Could you check a few things on this model? Use its own coordinates, in mm. Face numbers are marked on the shaded views. Give positions to 0.01 mm unless a question says otherwise; leave off trailing zeros. Write each loop counter-clockwise with the first axis right and the second up, starting at its lowest first coordinate (ties: lowest second). Pieces come first, ordered by that corner, then holes. Notation, with made-up numbers: (-9.75, 36) - (40.25, 36) arc R24 cw to (40.25, 48) - close; hole circle Ø5 at (71, -2). An arc over 180 degrees is marked (long way). Answer as a JSON object with one key per item and string values. Group by question number.
```python
from build123d import *

# Parameters (mm, degrees)
F3_DEPTH = 3.81
F4_R     = 1.27


# Not quite as in the source:
# - the program builds the solid bodies; features that only make, move or delete a surface that nothing else refers to are left out


with BuildPart() as f3:
    # F2 (on Front) → F3 (new body, symmetric)
    with BuildSketch(Plane.XZ):
        Polygon((67.4008423153, 47.9680152879), (42.0008423153, 47.9680152879), (33.6273413479, 18.6607656464), (59.0273413479, 18.6607656464), align=None)
    extrude(amount=F3_DEPTH, both=True)

    # F4
    f4_edges = [f3.edges().sort_by_distance(p)[0] for p in [
        (54.700842, -3.81, 47.968015),
        (63.214092, -3.81, 33.31439),
        (46.327341, -3.81, 18.660766),
        (63.214092, 3.81, 33.31439),
        (54.700842, 3.81, 47.968015),
        (46.327341, 3.81, 18.660766),
        (67.400842, 0, 47.968015),
        (59.027341, 0, 18.660766),
    ]]
    fillet(f4_edges, radius=F4_R)


solid = f3.part
```
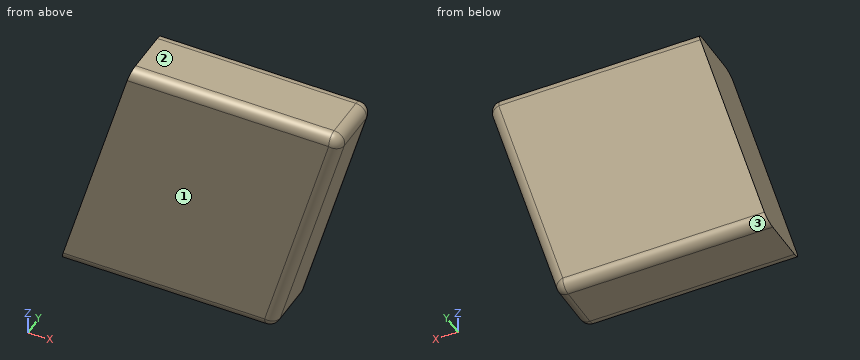
(1) I want a section at B-B, the plane x = 39.5. Please give me the cut outline in (y, z), and give its area (3 significant figures).
(2) I want a section at A-A, the plane y = -2. Please give me the cut outline in (x, z).
(3) I need wall thicknesses on L1, parallel to X at y = 2.5, z = 24; L2, parallel to Z at x = 52.5, y = -2.75; L3, parallel to Z at x = 55.5, y = 3.25. Which ranges of each line are inside material? Lowest first, please.
(4) Will these pins go through, and if not, where does the flat tip stop? P1, Ø3, axis at y = 0.5, z = 24, coming from the +X side; P2, Ø3, axis at y = -1, z = 34, coming from the +X side.
(5) If we mould it in two halves opening along Z, with no side actions, what happens to the marked faces 1, 2 and 3? For each: +Z half, -Z half, draft (parallel to the pull), parting line (faces both ways), or undercut.
Entries:
{
 "1": {"outline": "(-3.81, 19.93) arc R1.27 ccw to (-2.54, 18.66) - (2.54, 18.66) arc R1.27 ccw to (3.81, 19.93) - (3.81, 39.22) - (-3.81, 39.22) - close", "area": "156 mm^2"},
 "2": {"outline": "(33.63, 18.66) - (58.07, 18.66) arc R1.27 ccw to (59.29, 19.58) - (66.94, 46.35) arc R1.27 ccw to (65.72, 47.97) - (42, 47.97) - close"},
 "3": {"L1": "35.15 to 60.55", "L2": "18.68 to 47.95", "L3": "18.88 to 47.75"},
 "4": {"P1": "x = 60.98", "P2": "x = 63.84"},
 "5": {"face 1": "draft", "face 2": "+Z half", "face 3": "-Z half"}
}
